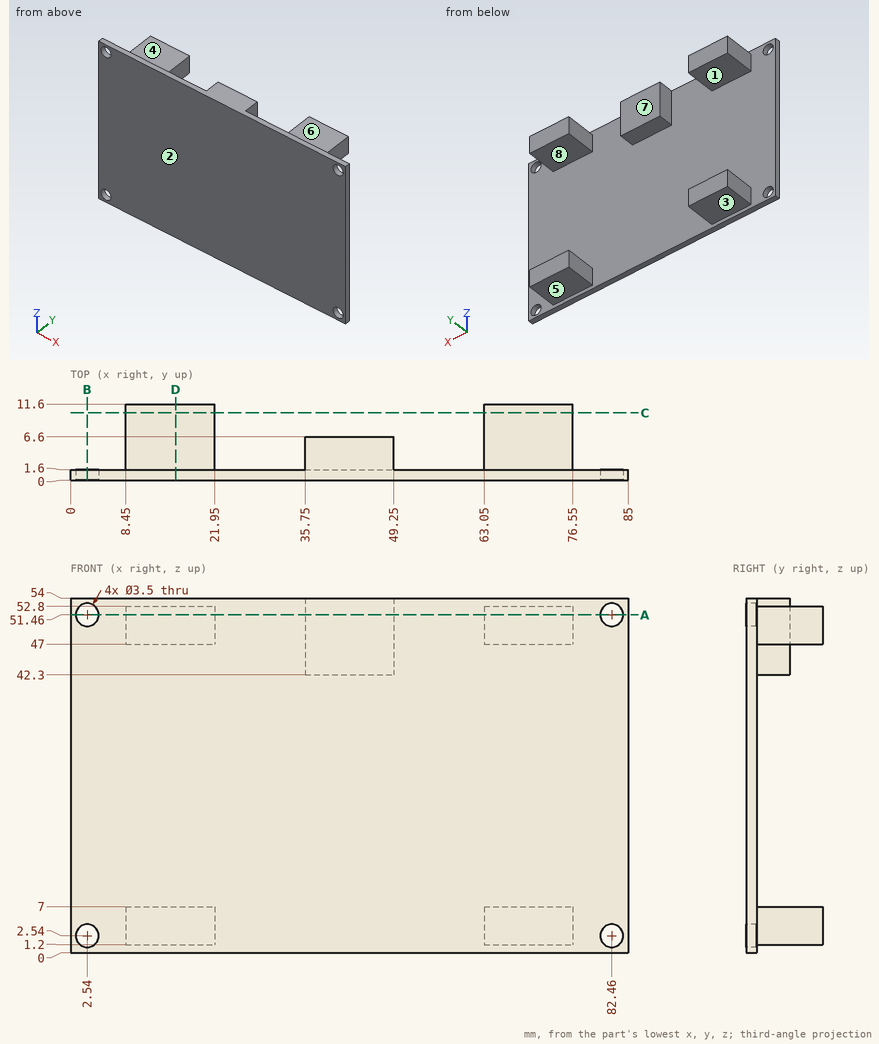
Here's the drawing with two shaded views (mm, measured from the low corner). I have some questions. A direction names the side the tool comes from. Coordinates: 2 decimals unless noted, no trailing zeros. Write each loop counter-clockwise with the first axis right and the second up, starting at its lowest first coordinate (ties: lowest second). Pieces come first, ordered by that corner, then holes. Notation, with made-up numbers: (-10, -14.75) -> (47, -14.75) arc R36 cw to (47, 20.25) -> close; hole circle Ø4 at (67, -37.5). An arc over 180 degrees is marked (long way). Write item = value, one per line. Start each with the question number.
(1) We'd pull the mould along Z, two halves only. Please class the marked faces 1, 2 and 3: released by +Z, released by -Z, zero draft, split by the parting line, or undercut.
(2) I want a section at A-A (z = 51.46). Please give me the cut outline in (x, y), plus the area to 3 significant figures.
(3) I want a section at C-C (y = 10.25). Please give me the cut outline in (x, z), plus the area to 3 significant figures.
(4) Which directions (+Z, -Z, +X, -X, +Y, -Y) give clear straight access to the entire face, cutting with the end or side of a thin tool? Please do the marked faces 4, 5, 6, 7 and 8.
(5) Will these pins go through, and if not, where does the flat tip stop? pin 1 (4.5 mm diameter, centred on y = 8.5, z = 5, fed in from -X); pin 2 (3 mm diameter, centred on x = 2.54, z = 51.46, fed in from -Y); pin 3 (1 mm diameter, centred on x = 65.5, y = 3, fed in from -Z); pin 4 (4 mm diameter, centred on x = 40.5, y = 4, fed in from -Z).
(6) I want a section at B-B (x = 2.54). Please give me the cut outline in (y, z).
(7) I need wall thicknesses on line 1 (Z direction, x = 2.54, y = 0.7); line 2 (X direction, y = 5.5, z = 49.5); line 3 (Z direction, x = 14.5, y = 3). Which ranges of each line are inside material? Lowest first, please. Write a range as [from, to].
(8) I want a section at D-D (x = 16). Please give me the cut outline in (y, z), plus the area to 3 significant figures.
Result set:
q1.face_1 = undercut
q1.face_2 = zero draft
q1.face_3 = released by -Z
q2.outline = (0, 0) -> (0.79, 0) -> (0.79, 1.6) -> (0, 1.6) -> close; (4.29, 0) -> (80.71, 0) -> (80.71, 1.6) -> (76.55, 1.6) -> (76.55, 11.6) -> (63.05, 11.6) -> (63.05, 1.6) -> (49.25, 1.6) -> (49.25, 6.6) -> (35.75, 6.6) -> (35.75, 1.6) -> (21.95, 1.6) -> (21.95, 11.6) -> (8.45, 11.6) -> (8.45, 1.6) -> (4.29, 1.6) -> close; (84.21, 0) -> (85, 0) -> (85, 1.6) -> (84.21, 1.6) -> close
q2.area = 462 mm2
q3.outline = (8.45, 1.2) -> (21.95, 1.2) -> (21.95, 7) -> (8.45, 7) -> close; (8.45, 47) -> (21.95, 47) -> (21.95, 52.8) -> (8.45, 52.8) -> close; (63.05, 1.2) -> (76.55, 1.2) -> (76.55, 7) -> (63.05, 7) -> close; (63.05, 47) -> (76.55, 47) -> (76.55, 52.8) -> (63.05, 52.8) -> close
q3.area = 313 mm2
q4.face_4 = +Z, -X, +Y
q4.face_5 = -Z, +X, -X, +Y
q4.face_6 = +Z, +X, +Y
q4.face_7 = +Z, -Z, +Y
q4.face_8 = +X, +Y
q5.pin_1 = 8.45
q5.pin_2 = through
q5.pin_3 = 1.2
q5.pin_4 = 42.3
q6.outline = (0, 0) -> (1.6, 0) -> (1.6, 0.79) -> (0, 0.79) -> close; (0, 4.29) -> (1.6, 4.29) -> (1.6, 49.71) -> (0, 49.71) -> close; (0, 53.21) -> (1.6, 53.21) -> (1.6, 54) -> (0, 54) -> close
q7.line_1 = [0, 0.79], [4.29, 49.71], [53.21, 54]
q7.line_2 = [8.45, 21.95], [35.75, 49.25], [63.05, 76.55]
q7.line_3 = [1.2, 7], [47, 52.8]
q8.outline = (0, 0) -> (1.6, 0) -> (1.6, 1.2) -> (11.6, 1.2) -> (11.6, 7) -> (1.6, 7) -> (1.6, 47) -> (11.6, 47) -> (11.6, 52.8) -> (1.6, 52.8) -> (1.6, 54) -> (0, 54) -> close
q8.area = 202 mm2
